Part model, mm, in its own coordinate system. A direction names the side the tool comes from. Give positions to 0.01 mm unless a question says otherwise; leave off trailing zeros. Write each loop counter-clockwise with the first axis right and the second up, starting at its lowest first coordinate (ties: lowest second). Pieces come first, ordered by that corner, then holes. Notation, with made-up numbers: M -17.75,42.5 L 18.25,42.5 A12 cw 18.25,60.5 Z; hole C 5,34 d5. An arc over 180 degrees is marked long. Answer as CSV lines item,"result". Start each with the question number.
Item 1: 3-axis set-ups, long thin cutter, end or side, ignore diameter. For faces 1 (the flat face through (0, 44, -46.758)), 2 (the flat face through (0, 92, 34.058)), 3 (the flat face through (0, 82.55, -37)): which of +Z, -Z, +X, -X, +Y, -Y reach the whole face in a straight line?
Item 2: Band-saw the part on A-A, the plane y = 51. List the corners of the cut face in (x, z) (3 decimals).
Item 3: Band-saw the part on D-D, the plane z = 0. List the corners of the cut face in (x, y).
Item 4: Two-plate mould, pull along Y, no slides. Class faces 4 (the flat face through (1, 0, -1)), 5 (the flat face through (0, 95.25, -42)), 6 (the flat face through (3.175, 65, -44)): +Y half, -Y half, draft (parallel to the pull), parting line (faces both ways), or undercut.
Item 5: Band-saw the part on C-C, the plane y = 93. List the corners of the cut face in (x, z) (3 decimals).
Item 6: Wall check: L1, parallel to Z at x = -2, y = 67; L2, parallel to Y at x = -13, z = 8; L3, parallel to X at y = 50.5, z = -41.5 (3 decimals). Give the ranges that are in metal, low to high. Write a range as from..to.
Item 7: Band-saw the part on B-B, the plane x = 0. List the corners of the cut face in (y, z).
Item 8: Pin check, flat tips, straight feed: pin 1 (3 mm diameter, centred on x = -1.5, y = 90.5, fed in from +Z); pin 2 (4.5 mm diameter, centred on y = 71, z = -43.5, fed in from +X) (3 decimals); pin 3 (10 mm diameter, centred on x = -34, z = 0.5, fed in from +Y). Stop position of each tip, or through.
from build123d import *

# Parameters (mm, degrees)
SKETCH1_R           = 50.8
BOSS_EXTRUDE1_DEPTH = 6.35
SKETCH9_W           = 6.35
SKETCH9_H           = 76.2
SKETCH9_W_2         = 8.636
SKETCH9_H_2         = 6.35
BOSS_EXTRUDE5_DEPTH = 3.175


with BuildPart() as part:
    # Sketch1 → Boss-Extrude1 (new body)
    with BuildSketch(Plane(origin=(0, 0, 0), x_dir=(1, 0, 0), z_dir=(0, 1, 0))):
        with Locations(Location((0, 0, 0), (0, 0, 270))):
            Circle(SKETCH1_R)
    extrude(amount=BOSS_EXTRUDE1_DEPTH)

    # Sketch9 → Boss-Extrude5 (add, symmetric)
    # profile 1 of 2: a face of its own
    with BuildSketch(Plane(origin=(0, 0, 0), x_dir=(0, 0, -1), z_dir=(1, 0, 0))):
        with Locations((43.583352, 44.45)):
            Rectangle(SKETCH9_W, SKETCH9_H)
    # profile 2 of 2: a face of its own
    with BuildSketch(Plane(origin=(0, 0, 0), x_dir=(0, 0, -1), z_dir=(1, 0, 0))):
        Polygon((34.058352, 82.55), (40.408352, 82.55), (46.758352, 82.55), (49.806352, 82.55), (49.806352, 101.6), (34.058352, 101.6), align=None)
        with Locations((42.440352, 92.075)):
            Rectangle(SKETCH9_W_2, SKETCH9_H_2, mode=Mode.SUBTRACT)
    boss_extrude5 = extrude(amount=BOSS_EXTRUDE5_DEPTH, both=True)

    # Mirror1: Boss-Extrude5 across plane
    add(boss_extrude5.mirror(Plane.XY))


solid = part.part
Output:
1,face 1,"-Z, +X, -X"
1,face 2,"+X, -X, +Y"
1,face 3,"+X, -X"
2,outline,"M -3.175,-46.758 L 3.175,-46.758 L 3.175,-40.408 L -3.175,-40.408 Z; M -3.175,40.408 L 3.175,40.408 L 3.175,46.758 L -3.175,46.758 Z"
3,outline,"M -50.8,0 L 50.8,0 L 50.8,6.35 L -50.8,6.35 Z"
4,face 4,"-Y half"
4,face 5,"undercut"
4,face 6,"draft"
5,outline,"M -3.175,-49.806 L 3.175,-49.806 L 3.175,-46.758 L -3.175,-46.758 Z; M -3.175,-38.122 L 3.175,-38.122 L 3.175,-34.058 L -3.175,-34.058 Z; M -3.175,34.058 L 3.175,34.058 L 3.175,38.122 L -3.175,38.122 Z; M -3.175,46.758 L 3.175,46.758 L 3.175,49.806 L -3.175,49.806 Z"
6,L1,"-46.76..-40.41, 40.41..46.76"
6,L2,"0..6.35"
6,L3,"-3.175..3.175"
7,outline,"M 0,-50.8 L 6.35,-50.8 L 6.35,-46.76 L 82.55,-46.76 L 82.55,-49.81 L 101.6,-49.81 L 101.6,-34.06 L 82.55,-34.06 L 82.55,-40.41 L 6.35,-40.41 L 6.35,40.41 L 82.55,40.41 L 82.55,34.06 L 101.6,34.06 L 101.6,49.81 L 82.55,49.81 L 82.55,46.76 L 6.35,46.76 L 6.35,50.8 L 0,50.8 Z; hole M 88.9,-46.76 L 95.25,-46.76 L 95.25,-38.12 L 88.9,-38.12 Z; hole M 88.9,38.12 L 95.25,38.12 L 95.25,46.76 L 88.9,46.76 Z"
8,pin 1,"z = 49.81"
8,pin 2,"x = 3.175"
8,pin 3,"y = 6.35"
